```python
from build123d import *

# Parameters (mm, degrees)
F1_DEPTH = 2.54
F3_DEPTH = 2.541
F4_DEPTH = 0.635
F5_DEPTH = 0.3175


with BuildPart() as f1:
    # F0 (on Top) → F1 (new body)
    with BuildSketch(Plane.XY):
        Polygon((11.43, 8.89), (0, 17.78), (-3.81, 8.89), (-3.81, 0), (6.35, -7.62), align=None)
    extrude(amount=F1_DEPTH)

    # F2 (on face) → F3 (cut, through all)
    with BuildSketch(Plane.XY.offset(2.54)):
        Polygon((-3.048, 6.140546), (2.421456, 13.172704), (-1.145524, 13.172704), (-3.048, 8.733594), align=None)
        Polygon((7.885093, 10.681801), (3.875184, 13.80062), (2.129282, 11.555889), (6.139191, 8.43707), align=None)
        Polygon((2.281741, -3.616306), (2.281741, 10.479143), (-2.531702, -0.006223), align=None)
        Polygon((8.186874, 0.94092), (5.686294, 1.710329), (5.39678, 0.769409), (7.89736, 0), align=None)
    extrude(amount=-F3_DEPTH, mode=Mode.SUBTRACT)

    # F2 (on face) → F4 (cut, symmetric)
    with BuildSketch(Plane.XY.offset(2.54)):
        Polygon((6.155309, 5.825708), (3.043741, 8.245816), (3.043741, -4.286889), align=None)
        Polygon((10.547025, 8.61141), (8.486579, 10.213979), (6.740677, 7.969248), (9.652572, 5.70444), align=None)
        Polygon((-3.048, 0.69555), (1.661459, 10.954402), (-3.048, 4.899384), align=None)
    extrude(amount=F4_DEPTH, both=True, mode=Mode.SUBTRACT)

    # F2 (on face) → F5 (cut, symmetric)
    with BuildSketch(Plane.XY.offset(2.54)):
        Polygon((7.51598, -1.239484), (5.015401, -0.470075), (3.733805, -4.635261), (6.234384, -5.40467), align=None)
        Polygon((9.376229, 4.806324), (6.875649, 5.575733), (5.898628, 2.400413), (8.399207, 1.631004), align=None)
        Polygon((3.70279, 13.934704), (0.311483, 16.572387), (-0.818953, 13.934704), align=None)
    extrude(amount=F5_DEPTH, both=True, mode=Mode.SUBTRACT)


solid = f1.part
```
Geometry check sheet. Reference: the model listing, model coordinates, mm. A direction names the side the tool comes from. Round coordinates to 2 decimals unless told otherwise and drop trailing zeros. Order: outer loops, then holes, each group sorted by start corner. A loop starts at its lowest first (then second) coordinate and runs counter-clockwise, first axis right, second up. Notation, with made-up numbers: (31, 38.5) - (75, 38.5) arc R22 ccw to (75, 52.5) - close; hole circle Ø8 at (87, -18.5). An arc over 180 degrees is marked (long way). Use a Markdown table: item, result. Add a question column.
1) Set-up check for faces 1 (the flat face through (-0.35, 9.61, 1.29)), 2 (the flat face through (4, 3, 1.905)): record each of +Z, -Z, +X, -X, +Y, -Y from which the full face is reachable in a straight line by a thin tool's end or side.
2) Gauge pin test, flat ends, axial feed: P1, Ø1.3, axis at x = 1.5, z = 1.5, coming from the -Y side; P2, Ø1.3, axis at x = 0.5, y = 15, coming from the +Z side; P3, Ø1.3, axis at y = 8, z = 1, coming from the +X side. Record the tip position at first contact, or that the pin passes through.
3) Mould release check, pull along Y, two halves, no side actions. Record for faces 3 (the flat face through (1, 15, 2.222)), 4 (the flat face through (5.8, 13.27, 1.25)), 5 (the flat face through (4, 5, 0)): released by +Y, released by -Y, zero draft, split by the parting line, or undercut.
4) Section check A-A (y = 7). Record the cut outline in (x, z) (1 decimal), then the cut area to 3 significant figures.
5) Thickness scan on line 1 along Y through (x, z) = (6.25, 0.3) (3 decimals); line 2 along Y through (x, z) = (1.5, 0.75); line 3 along X through (y, z) = (11, 2.45). Record the ranges inside material, lowest first.
6) Section check D-D (x = 0.75). Count the separate pieces of the cut face and the enclosed holes in it, then the cut area to 3 significant figures.
7) Section check B-B (z = 1.15). Record the cut outline in (x, y).
Established:
| question | item | result |
|---|---|---|
| 1 | face 1 | +Z, -Z |
| 1 | face 2 | +Z |
| 2 | P1 | y = -4.47 |
| 2 | P2 | z = 2.22 |
| 2 | P3 | x = 11.36 |
| 3 | face 3 | undercut |
| 3 | face 4 | released by +Y |
| 3 | face 5 | zero draft |
| 4 | outline | (-3.8, 0) - (-3, 0) - (-3, 2.5) - (-3.8, 2.5) - close; (-2.4, 0) - (0.7, 0) - (0.7, 2.5) - (-0.2, 2.5) - (-0.2, 1.9) - (-1.4, 1.9) - (-1.4, 2.5) - (-2.4, 2.5) - close; (2.3, 0) - (10.8, 0) - (10.8, 2.5) - (10.1, 2.5) - (10.1, 1.9) - (8, 1.9) - (8, 2.5) - (4.6, 2.5) - (4.6, 1.9) - (3, 1.9) - (3, 2.5) - (2.3, 2.5) - close |
| 4 | area | 28.3 mm2 |
| 5 | line 1 | -7.545 to 0.507, 1.537 to 8.58, 11.954 to 12.919 |
| 5 | line 2 | -3.98 to -3.03, 8.78 to 11.99, 13.17 to 16.61 |
| 5 | line 3 | -2.91 to -2.08, 0.73 to 2.84, 7.48 to 8.72 |
| 6 | separate pieces | 3 |
| 6 | enclosed holes | 0 |
| 6 | area | 21.3 mm2 |
| 7 | outline | (-3.81, 0) - (6.35, -7.62) - (11.43, 8.89) - (0, 17.78) - (-3.81, 8.89) - close; hole (-3.05, 6.14) - (2.42, 13.17) - (-1.15, 13.17) - (-3.05, 8.73) - close; hole (-2.53, -0.01) - (2.28, -3.62) - (2.28, 10.48) - close; hole (2.13, 11.56) - (6.14, 8.44) - (7.89, 10.68) - (3.88, 13.8) - close; hole (5.4, 0.77) - (7.9, 0) - (8.19, 0.94) - (5.69, 1.71) - close |
